from build123d import *

# Parameters (mm, degrees)
ESQUISSE1_W             = 98
ESQUISSE1_H             = 98
BOSS_EXTRU_1_DEPTH      = 47.5
BOSS_EXTRU_1_TAPER      = 20
ESQUISSE2_R             = 25
ENL_V_MAT_EXTRU_1_DEPTH = 147.50682578
ENL_V_MAT_EXTRU_4_DEPTH = 169.026783579
CONG_1_R                = 15
ESQUISSE4_R             = 35
ENL_V_MAT_EXTRU_5_DEPTH = 10
ENL_V_START             = -10
ESQUISSE5_R             = 35
ENL_V_MAT_EXTRU_6_DEPTH = 10
BOSS_EXTRU_2_DEPTH      = 10
CONG_2_R                = 5
ENL_V_MAT_EXTRU_7_DEPTH = 10


with BuildPart() as part:
    # Esquisse1 → Boss.-Extru.1 (new body)
    with BuildSketch(Plane.XY):
        with Locations((49, 49)):
            Rectangle(ESQUISSE1_W, ESQUISSE1_H)
    boss_extru_1 = extrude(amount=BOSS_EXTRU_1_DEPTH, taper=BOSS_EXTRU_1_TAPER)

    # Esquisse2 → Enlèv. mat.-Extru.1 (cut, through all)
    with BuildSketch(Plane(origin=(0, 0, 0), x_dir=(-1, 0, 0), z_dir=(0, 0, -1))):
        with Locations((-49, 49)):
            Circle(ESQUISSE2_R)
    enl_v_mat_extru_1 = extrude(amount=-ENL_V_MAT_EXTRU_1_DEPTH, mode=Mode.SUBTRACT)

    # Symétrie1: Boss.-Extru.1, Enlèv. mat.-Extru.1 across plane
    add(boss_extru_1.mirror(Plane.XY.offset(47.5)))
    add(enl_v_mat_extru_1.mirror(Plane.XY.offset(47.5)), mode=Mode.SUBTRACT)

    # Esquisse3 → Enlèv. mat.-Extru.4 (cut, through all)
    with BuildSketch(Plane.XY.offset(95)):
        with BuildLine():
            ThreePointArc((74, 49), (66.67766953, 31.32233047), (49, 24))
            Line((49, 24), (49, 0))
            Line((49, 0), (98, 0))
            Line((98, 0), (98, 49))
            Line((98, 49), (74, 49))
        make_face()
    extrude(amount=-ENL_V_MAT_EXTRU_4_DEPTH, mode=Mode.SUBTRACT)

    # Congé1
    cong_1_edges = [part.edges().sort_by_distance(p)[0] for p in [
        (33.144293064, 17.288586128, 47.5),
        (17.288586128, 49, 47.5),
        (80.711413872, 64.855706936, 47.5),
        (49, 80.711413872, 47.5),
    ]]
    fillet(cong_1_edges, radius=CONG_1_R)

    # Esquisse4 → Enlèv. mat.-Extru.5 (cut)
    with BuildSketch(Plane.XY.offset(95)):
        with Locations((49, 49)):
            Circle(ESQUISSE4_R)
    extrude(amount=-ENL_V_MAT_EXTRU_5_DEPTH, mode=Mode.SUBTRACT)

    # Esquisse5 → Enlèv. mat.-Extru.6 (cut)
    with BuildSketch(Plane(origin=(0, 0, 0), x_dir=(-1, 0, 0), z_dir=(0, 0, -1)).offset(ENL_V_START)):
        with Locations((-49, 49)):
            Circle(ESQUISSE5_R)
    extrude(amount=ENL_V_MAT_EXTRU_6_DEPTH, mode=Mode.SUBTRACT)

    # Esquisse6 → Boss.-Extru.2 (add)
    with BuildSketch(Plane(origin=(0, 0, 0), x_dir=(-1, 0, 0), z_dir=(0, 0, -1))):
        Polygon((-98, 49), (-98, 98), (0, 98), (0, 0), (-49, 0), (-49, 3), (-3, 3), (-3, 95), (-95, 95), (-95, 49), align=None)
    extrude(amount=BOSS_EXTRU_2_DEPTH)

    # Congé2
    cong_2_edges = [part.edges().sort_by_distance(p)[0] for p in [
        (98, 73.5, 0),
        (0, 49, 0),
        (24.5, 0, 0),
        (49, 98, 0),
    ]]
    fillet(cong_2_edges, radius=CONG_2_R)

    # Esquisse7 → Enlèv. mat.-Extru.7 (cut)
    with BuildSketch(Plane(origin=(0, 0, 0), x_dir=(-1, 0, 0), z_dir=(0, 0, -1))):
        with BuildLine():
            Line((-87.537319575, 91.779960262), (-76.930717857, 81.173358544))
            ThreePointArc((-76.930717857, 81.173358544), (-76.930717857, 76.930717857), (-81.173358544, 76.930717857))
            Line((-81.173358544, 76.930717857), (-91.779960262, 87.537319575))
            ThreePointArc((-91.779960262, 87.537319575), (-91.779960262, 91.779960262), (-87.537319575, 91.779960262))
        make_face()
        with BuildLine():
            Line((-6.220039738, 87.537319575), (-16.826641456, 76.930717857))
            ThreePointArc((-16.826641456, 76.930717857), (-21.069282143, 76.930717857), (-21.069282143, 81.173358544))
            Line((-21.069282143, 81.173358544), (-10.462680425, 91.779960262))
            ThreePointArc((-10.462680425, 91.779960262), (-6.220039738, 91.779960262), (-6.220039738, 87.537319575))
        make_face()
        with BuildLine():
            Line((-10.462680425, 6.220039738), (-21.069282143, 16.826641456))
            ThreePointArc((-21.069282143, 16.826641456), (-21.069282143, 21.069282143), (-16.826641456, 21.069282143))
            Line((-16.826641456, 21.069282143), (-6.220039738, 10.462680425))
            ThreePointArc((-6.220039738, 10.462680425), (-6.220039738, 6.220039738), (-10.462680425, 6.220039738))
        make_face()
    extrude(amount=-ENL_V_MAT_EXTRU_7_DEPTH, mode=Mode.SUBTRACT)


solid = part.part
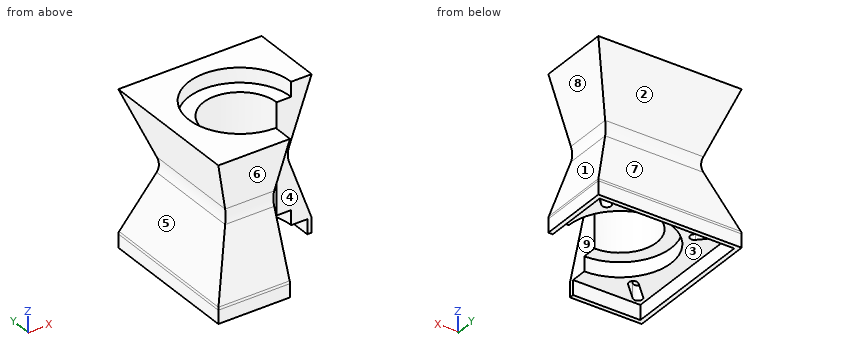
Could you check a few things on this model? Use its own coordinates, in mm. Face numbers are marked on the shaded views. A direction names the side the tool comes from. Coordinates: 2 decimals unless noted, no trailing zeros. Loops run counter-clockwise (first coordinate to the right, second up) from the corner with the lowest first, then second, coordinate; pieces in that order, holes last.
1. Imagine slicing it at C-C (z = 89.5). Please give me the cut outline in (x, y).
2. Imagine slicing it at B-B (x = 90). Please give me the cut outline in (y, z).
3. We'd pull the mould along Y, two halves only. Please class the marked faces 1, 2, 3 and 4: released by +Y, released by -Y, zero draft, split by the parting line, or undercut.
4. For the marked faces 5, 6, 7, 8 and 9, which set-ups out of +Z, -Z, +X, -X, +Y, -Y let a thin tool reach every point of the face, with its end or its side?
5. Imagine slicing it at A-A (y = 63). Please give me the cut outline in (x, z).
6. For P1, Ø1, axis at y = 39.5, z = 66, coming from the +X side; P2, Ø21, axis at x = 62.5, y = 55, coming from the -Z side; P3, Ø5, axis at x = 12, y = 16, coming from the -Z side, each with a flat end and sliding along its axis, tell me the tip position at first contact or that it passes through.
7. I need wall thicknesses on L1, parallel to X at y = 65.5, z = -2; L2, parallel to Y at x = 75, z = 17. Which ranges of each line are inside material? Lowest first, please.
8. Imagine slicing it at D-D (z = 28). Please give me the cut outline in (x, y), and give its area (3 significant figures).
Computed values:
1. outline: (2, 2) - (49, 2) - (49, 14) arc R35 cw (long way) to (84, 49) - (96, 49) - (96, 96) - (2, 96) - close
2. outline: (49, 0) - (85.76, 0) - (85.76, 10) - (92.64, 10) - (92.64, 0) - (95, 0) - (95, -10) - (98, -10) - (98, -0.88) arc R5 ccw to (97.7, 0.83) - (90, 21.98) - (49, 21.98) - close; (49, 73.02) - (90, 73.02) - (98, 95) - (49, 95) - close
3. face 1: zero draft
3. face 2: released by +Y
3. face 3: undercut
3. face 4: released by -Y
4. face 5: -X, +Y, -Y
4. face 6: +X, -X, -Y
4. face 7: +X, -X, +Y
4. face 8: +X, +Y, -Y
4. face 9: +Z, -Z, +X, -Y
5. outline: (0, -10) - (3, -10) - (3, 0) - (16.92, 0) - (16.92, 10) - (28.29, 10) - (28.29, 85) - (16.92, 85) - (16.92, 95) - (0, 95) - (15.42, 52.63) arc R15 cw to (15.42, 42.37) - (0.3, 0.83) arc R5 ccw to (0, -0.88) - close; (69.71, 10) - (81.08, 10) - (81.08, 0) - (95, 0) - (95, -10) - (98, -10) - (98, -0.88) arc R5 ccw to (97.7, 0.83) - (82.58, 42.37) arc R15 cw to (82.58, 52.63) - (98, 95) - (81.08, 95) - (81.08, 85) - (69.71, 85) - close
6. P1: stops at x = 26.09
6. P2: stops at z = 10
6. P3: stops at z = 0
7. L1: x = 0 to 3, 95 to 98
7. L2: y = 49 to 91.81
8. outline: (10.19, 10.19) - (49, 10.19) - (49, 24) arc R25 cw (long way) to (74, 49) - (87.81, 49) - (87.81, 87.81) - (10.19, 87.81) - close
8. area: 3,050 mm2
